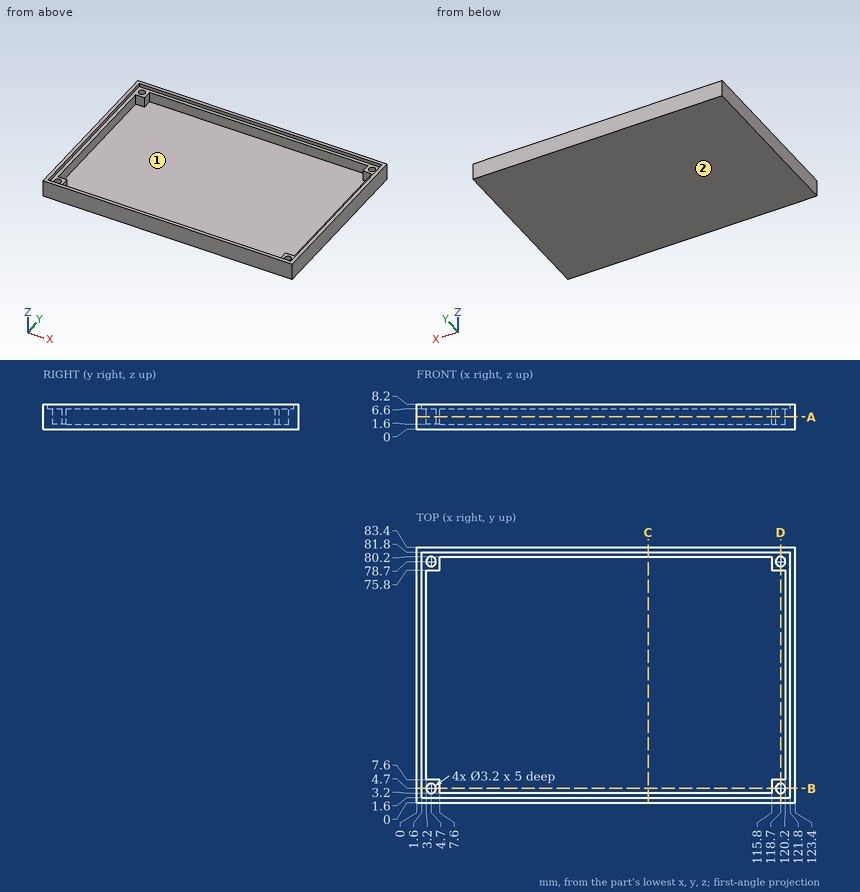
Drawing for the job (mm, zero at the part's lowest x, y, z). Round coordinates to 2 decimals unless told otherwise and drop trailing zeros. Write each loop counter-clockwise with the first axis right and the second up, starting at its lowest first coordinate (ties: lowest second). Pieces come first, ordered by that corner, then holes. Notation, with made-up numbers: (-26, -32) - (11, -32) arc R12 cw to (11, -10) - close; hole circle Ø9 at (7, -28). An arc over 180 degrees is marked (long way). Return JSON: item names as keys, results as strings. Group by question number.
Item 1: Band-saw the part on D-D on x = 118.7. List the corners of the cut face in (y, z), plus the area to 3 significant figures.
Item 2: Flat gauge pins, fed straight in: pin 1 Ø2.5 at (x, y) = (4.7, 78.7) entering from +Z; pin 2 Ø2.5 at (x, y) = (5, 5.5) entering from +Z. Where does each tip first touch, or does it go through?
Item 3: Band-saw the part on B-B on y = 4.7. List the corners of the cut face in (x, z).
Item 4: Band-saw the part on A-A on z = 4. List the corners of the cut face in (x, y).
Item 5: Probe probe 1 along Y at (x, z) = (118.7, 4.55); probe 2 along X at (y, z) = (43, 6.5); probe 3 along X at (y, z) = (75.5, 7.75). List the from-to ranges inside material, lowest first.
Item 6: Mould opens along X. For the marked faces 1 and 2 say: +X half, -X half, draft (parallel to the pull), parting line (faces both ways), or undercut.
Item 7: Band-saw the part on C-C on x = 75.5. List the corners of the cut face in (y, z), plus the area to 3 significant figures.
Resolved:
{
 "1": {"outline": "(0, 0) - (83.4, 0) - (83.4, 8.2) - (81.8, 8.2) - (81.8, 6.6) - (80.3, 6.6) - (80.3, 1.6) - (77.1, 1.6) - (77.1, 6.6) - (75.8, 6.6) - (75.8, 1.6) - (7.6, 1.6) - (7.6, 6.6) - (6.3, 6.6) - (6.3, 1.6) - (3.1, 1.6) - (3.1, 6.6) - (1.6, 6.6) - (1.6, 8.2) - (0, 8.2) - close", "area": "183 mm²"},
 "2": {"pin 1": "stops at z = 1.6", "pin 2": "stops at z = 6.6"},
 "3": {"outline": "(0, 0) - (123.4, 0) - (123.4, 8.2) - (121.8, 8.2) - (121.8, 6.6) - (120.3, 6.6) - (120.3, 1.6) - (117.1, 1.6) - (117.1, 6.6) - (115.8, 6.6) - (115.8, 1.6) - (7.6, 1.6) - (7.6, 6.6) - (6.3, 6.6) - (6.3, 1.6) - (3.1, 1.6) - (3.1, 6.6) - (1.6, 6.6) - (1.6, 8.2) - (0, 8.2) - close"},
 "4": {"outline": "(0, 0) - (123.4, 0) - (123.4, 83.4) - (0, 83.4) - close; hole circle Ø3.2 at (4.7, 4.7); hole circle Ø3.2 at (4.7, 78.7); hole (3.2, 7.6) - (7.6, 7.6) - (7.6, 3.2) - (115.8, 3.2) - (115.8, 7.6) - (120.2, 7.6) - (120.2, 75.8) - (115.8, 75.8) - (115.8, 80.2) - (7.6, 80.2) - (7.6, 75.8) - (3.2, 75.8) - close; hole circle Ø3.2 at (118.7, 4.7); hole circle Ø3.2 at (118.7, 78.7)"},
 "5": {"probe 1": "y = 0 to 3.1, 6.3 to 7.6, 75.8 to 77.1, 80.3 to 83.4", "probe 2": "x = 0 to 3.2, 120.2 to 123.4", "probe 3": "x = 0 to 1.6, 121.8 to 123.4"},
 "6": {"face 1": "undercut", "face 2": "draft"},
 "7": {"outline": "(0, 0) - (83.4, 0) - (83.4, 8.2) - (81.8, 8.2) - (81.8, 6.6) - (80.2, 6.6) - (80.2, 1.6) - (3.2, 1.6) - (3.2, 6.6) - (1.6, 6.6) - (1.6, 8.2) - (0, 8.2) - close", "area": "171 mm²"}
}
